Read the model definition and answer for the solid it produces. Units are mm, in the model's axes. Face numbers are marked on the shaded views. A direction names the side the tool comes from. Give positions to 0.01 mm unless a question says otherwise; leave off trailing zeros. Loops run counter-clockwise (first coordinate to the right, second up) from the corner with the lowest first, then second, coordinate; pieces in that order, holes last. Notation, with made-up numbers: (-0.5, 72.5) - (34.5, 72.5) arc R25 cw to (34.5, 109.5) - close; hole circle Ø1 at (20.25, 48). An arc over 180 degrees is marked (long way). Put each result on its own line as item: value. Start each with the question number.
1. For the marked faces 1, 2 and 3, determine the directions among +Z, -Z, +X, -X, +Y, -Y from which every point of the face is accessible in a straight line to the end or side of a thin tool.
2. A cutting plane is placed at B-B, the plane x = 15.5. Determine the outline of the cut face in (y, z).
3. A cutting plane is placed at C-C, the plane y = 9.5. Determine the outline of the cut face in (x, z).
4. Consider L1, parallel to Y at x = 10, z = 0.75; L2, parallel to Z at x = -11, y = -2; L3, parallel to Y at x = 7.5, z = -8. Determine where each line is inside the solid, lowest interval first. Write a range as from..to.
5. Given pin 1 Ø6 at (x, z) = (9, -9.5) entering from +Y; pin 2 Ø1.5 at (x, y) = (6, 5.5) entering from -Z; pin 3 Ø0.5 at (y, z) = (0, 0.5) entering from +X, each flat-ended and moving along its own axis, determine where each tip first touches the part or whether it passes through.
6. A cutting plane is placed at D-D, the plane z = -3.75. Determine the outline of the cut face in (x, y).
7. A cutting plane is placed at A-A, the plane x = -10. Determine the outline of the cut face in (y, z).
```python
from build123d import *

# Parameters (mm, degrees)
F0_W         = 26
F0_H         = 38
F0_R         = 1.5
F1_DEPTH     = 3
F2_W         = 26
F2_H         = 8
F3_DEPTH     = 20
F5_DEPTH     = 5
F6_T1_DEPTH  = 3
F6_T3_DEPTH  = 18
F6_T5_DEPTH  = 19
F6_T7_DEPTH  = 13
F6_T9_DEPTH  = 41
F6_T11_DEPTH = 33
F6_T13_DEPTH = 34
F6_T15_DEPTH = 4
F6_T17_DEPTH = 8
F6_S21_W     = 2.04
F6_S21_H     = 2.04
F6_T22_DEPTH = 2.04
F6_S27_W     = 2.04
F6_S27_H     = 2.04
F6_T28_DEPTH = 2.04
F6_S33_W     = 2.04
F6_S33_H     = 2.04
F6_T34_DEPTH = 2.04
F6_T38_ANGLE = 90


# Not quite as in the source:
# - a fillet or chamfer that OpenCascade refuses, or shapes differently, is made with other operations: its cross-section is extruded or revolved along the edge and cut away or added


with BuildPart() as f1:
    # F0 (on Top) → F1 (new body)
    with BuildSketch(Plane.XY):
        Rectangle(F0_W, F0_H)
        with Locations((-10, 9.5)):
            Circle(F0_R, mode=Mode.SUBTRACT)
        with Locations((10, 9.5)):
            Circle(F0_R, mode=Mode.SUBTRACT)
    extrude(amount=F1_DEPTH)

    # F2 (on face) → F3 (join)
    with BuildSketch(Plane(origin=(0, 0, 0), x_dir=(1, 0, 0), z_dir=(0, 0, -1))):
        with Locations((0, 15)):
            Rectangle(F2_W, F2_H)
    extrude(amount=F3_DEPTH)

    # F4 (on face) → F5 (join)
    with BuildSketch(Plane.YZ.offset(13)):
        Polygon((-11, -20), (-11, 0), (-11, 3), (-19, 3), (-19, -20), align=None)
    extrude(amount=F5_DEPTH)

    # F6: fillet of radius 2 on 12 edges, made by hand

    # F6_s2 → F6_t1 (join)
    with BuildSketch(Plane.XY):
        with BuildLine():
            ThreePointArc((15, -11), (13.5857864376, -10.4142135624), (13, -9))
            Line((13, -9), (13, -11))
            Line((13, -11), (15, -11))
        make_face()
    extrude(amount=F6_T1_DEPTH)

    # F6_s4 → F6_t3 (cut)
    with BuildSketch(Plane.XY.offset(-18)):
        with BuildLine():
            ThreePointArc((-11, -11), (-12.4142135624, -11.5857864376), (-13, -13))
            Line((-13, -13), (-13, -11))
            Line((-13, -11), (-11, -11))
        make_face()
    extrude(amount=F6_T3_DEPTH, mode=Mode.SUBTRACT)

    # F6_s6 → F6_t5 (cut)
    with BuildSketch(Plane.XY.offset(-18)):
        with BuildLine():
            ThreePointArc((-11, -19), (-12.4142135624, -18.4142135624), (-13, -17))
            Line((-13, -17), (-13, -19))
            Line((-13, -19), (-11, -19))
        make_face()
    extrude(amount=F6_T5_DEPTH, mode=Mode.SUBTRACT)

    # F6_s8 → F6_t7 (cut)
    with BuildSketch(Plane.XY.offset(-5)):
        with BuildLine():
            ThreePointArc((13, 17), (12.4142135624, 18.4142135624), (11, 19))
            Line((11, 19), (13, 19))
            Line((13, 19), (13, 17))
        make_face()
        with BuildLine():
            ThreePointArc((-11, 19), (-12.4142135624, 18.4142135624), (-13, 17))
            Line((-13, 17), (-13, 19))
            Line((-13, 19), (-11, 19))
        make_face()
    extrude(amount=F6_T7_DEPTH, mode=Mode.SUBTRACT)

    # F6_s10 → F6_t9 (cut)
    with BuildSketch(Plane.XZ.offset(-24)):
        with BuildLine():
            ThreePointArc((-11, 3), (-12.4142135624, 2.4142135624), (-13, 1))
            Line((-13, 1), (-13, 3))
            Line((-13, 3), (-11, 3))
        make_face()
    extrude(amount=F6_T9_DEPTH, mode=Mode.SUBTRACT)

    # F6_s12 → F6_t11 (cut)
    with BuildSketch(Plane.XZ.offset(-24)):
        with BuildLine():
            ThreePointArc((13, 1), (12.4142135624, 2.4142135624), (11, 3))
            Line((11, 3), (13, 3))
            Line((13, 3), (13, 1))
        make_face()
    extrude(amount=F6_T11_DEPTH, mode=Mode.SUBTRACT)

    # F6_s14 → F6_t13 (cut)
    with BuildSketch(Plane.YZ.offset(-11)):
        with BuildLine():
            ThreePointArc((-13, -20), (-11.5857864376, -19.4142135624), (-11, -18))
            Line((-11, -18), (-11, -20))
            Line((-11, -20), (-13, -20))
        make_face()
        with BuildLine():
            ThreePointArc((-19, -18), (-18.4142135624, -19.4142135624), (-17, -20))
            Line((-17, -20), (-19, -20))
            Line((-19, -20), (-19, -18))
        make_face()
        with BuildLine():
            ThreePointArc((-19, 1), (-18.4142135624, 2.4142135624), (-17, 3))
            Line((-17, 3), (-19, 3))
            Line((-19, 3), (-19, 1))
        make_face()
    extrude(amount=F6_T13_DEPTH, mode=Mode.SUBTRACT)

    # F6_s16 → F6_t15 (cut)
    with BuildSketch(Plane.XZ.offset(13)):
        with BuildLine():
            ThreePointArc((-11, -20), (-12.4142135624, -19.4142135624), (-13, -18))
            Line((-13, -18), (-13, -20))
            Line((-13, -20), (-11, -20))
        make_face()
    extrude(amount=F6_T15_DEPTH, mode=Mode.SUBTRACT)

    # F6_s18 → F6_t17 (cut)
    with BuildSketch(Plane.YZ.offset(15)):
        with BuildLine():
            ThreePointArc((-11, 1), (-11.5857864376, 2.4142135624), (-13, 3))
            Line((-13, 3), (-11, 3))
            Line((-11, 3), (-11, 1))
        make_face()
    extrude(amount=F6_T17_DEPTH, mode=Mode.SUBTRACT)


with BuildPart() as f6_tool20:
    # F6_s21 → F6_t22 (new body)
    with BuildSketch(Plane.XY.offset(-18)):
        with Locations((-12.02, -11.98)):
            Rectangle(F6_S21_W, F6_S21_H)
    extrude(amount=-F6_T22_DEPTH)

    # F6_s23 → F6_t24 (revolve, cut)
    with BuildSketch(Plane(origin=(-11, -13, -18), x_dir=(0.7071067812, -0.7071067812, 0), z_dir=(0.7071067812, 0.7071067812, 0))):
        with BuildLine():
            ThreePointArc((0, -2), (2, 0), (0, 2))
            Line((0, 2), (0, -2))
        make_face()
    revolve(axis=Axis((-11, -13, -18), (0, 0, -1)), mode=Mode.SUBTRACT)


with BuildPart() as f1_1:
    add(f1.part)

    # F6_t19: cut F6_tool20
    add(f6_tool20.part, mode=Mode.SUBTRACT)


with BuildPart() as f6_tool26:
    # F6_s27 → F6_t28 (new body)
    with BuildSketch(Plane.XZ.offset(17)):
        with Locations((-12.02, 2.02)):
            Rectangle(F6_S27_W, F6_S27_H)
    extrude(amount=F6_T28_DEPTH)

    # F6_s29 → F6_t30 (revolve, cut)
    with BuildSketch(Plane(origin=(-11, -17, 1), x_dir=(0.7071067812, 0, -0.7071067812), z_dir=(-0.7071067812, 0, -0.7071067812))):
        with BuildLine():
            ThreePointArc((0, -2), (2, 0), (0, 2))
            Line((0, 2), (0, -2))
        make_face()
    revolve(axis=Axis((-11, -17, 1), (0, -1, 0)), mode=Mode.SUBTRACT)


with BuildPart() as f1_2:
    add(f1_1.part)

    # F6_t25: cut F6_tool26
    add(f6_tool26.part, mode=Mode.SUBTRACT)


with BuildPart() as f6_tool32:
    # F6_s33 → F6_t34 (new body)
    with BuildSketch(Plane.XZ.offset(17)):
        with Locations((-12.02, -19.02)):
            Rectangle(F6_S33_W, F6_S33_H)
    extrude(amount=F6_T34_DEPTH)

    # F6_s35 → F6_t36 (revolve, cut)
    with BuildSketch(Plane(origin=(-11, -17, -18), x_dir=(0.7071067812, 0, 0.7071067812), z_dir=(0.7071067812, 0, -0.7071067812))):
        with BuildLine():
            ThreePointArc((0, -2), (2, 0), (0, 2))
            Line((0, 2), (0, -2))
        make_face()
    revolve(axis=Axis((-11, -17, -18), (0, -1, 0)), mode=Mode.SUBTRACT)


with BuildPart() as f1_3:
    add(f1_2.part)

    # F6_t31: cut F6_tool32
    add(f6_tool32.part, mode=Mode.SUBTRACT)

    # F6_s37 → F6_t38 (revolve, cut)
    with BuildSketch(Plane.YZ.offset(15)):
        with BuildLine():
            ThreePointArc((-11, 1), (-11.5857864376, 2.4142135624), (-13, 3))
            Line((-13, 3), (-11, 3))
            Line((-11, 3), (-11, 1))
        make_face()
    revolve(axis=Axis((15, -9, 3), (0, 0, -1)), revolution_arc=F6_T38_ANGLE, mode=Mode.SUBTRACT)


solid = f1_3.part
```
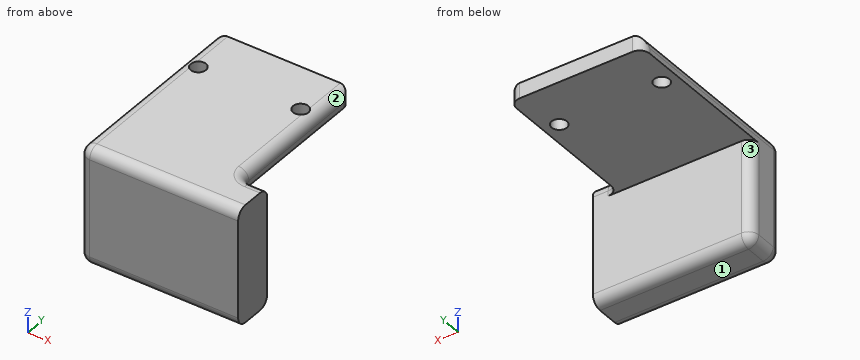
Return value:
1. face 1: -Z, +X, -X, +Y, -Y
1. face 2: +Z, +X, +Y
1. face 3: -Z, -X, +Y
2. outline: (-19, -18) arc R2 ccw to (-17, -20) - (-13, -20) arc R2 ccw to (-11, -18) - (-11, 1) arc R2 ccw to (-13, 3) - (-17, 3) arc R2 ccw to (-19, 1) - close
3. outline: (-13, 0) - (-11.5, 0) - (-11.5, 2.94) arc R2 ccw to (-13, 1) - close; (-8.5, 0) - (8.5, 0) - (8.5, 3) - (-8.5, 3) - close; (11.5, 0) - (13, 0) - (13, 1) arc R2 ccw to (11.5, 2.94) - close
4. L1: y = -19..8, 11..19
4. L2: z = 0..3
4. L3: y = -19..-11
5. pin 1: stops at y = -11
5. pin 2: stops at z = 0
5. pin 3: stops at x = 13
6. outline: (-13, -17) arc R2 ccw to (-11, -19) - (18, -19) - (18, -11) - (-11, -11) arc R2 ccw to (-13, -13) - close
7. outline: (-19, -18) arc R2 ccw to (-17, -20) - (-13, -20) arc R2 ccw to (-11, -18) - (-11, 0) - (8, 0) - (8, 3) - (-17, 3) arc R2 ccw to (-19, 1) - close; (11, 0) - (19, 0) - (19, 3) - (11, 3) - close
